from build123d import *

# Parameters (mm, degrees)
SKETCH1_W           = 13
SKETCH1_H           = 120
BOSS_EXTRUDE1_DEPTH = 9
SKETCH2_W           = 4.9
SKETCH2_H           = 6.8
BOSS_EXTRUDE2_DEPTH = 9
LPATTERN1_COUNT     = 4
LPATTERN1_PITCH     = 32
SKETCH3_W           = 4.8
SKETCH3_H           = 4.8
BOSS_EXTRUDE3_DEPTH = 9
LPATTERN2_COUNT     = 3
LPATTERN2_PITCH     = 32
SKETCH4_R           = 1.5
CUT_EXTRUDE1_DEPTH  = 9.6
CUT_EXTRUDE2_START  = -9.6
SKETCH5_R           = 1.5
CUT_EXTRUDE2_DEPTH  = 9.6
SKETCH6_W           = 13
SKETCH6_H           = 1.6
BOSS_EXTRUDE4_DEPTH = 3.7
LPATTERN3_COUNT     = 8
LPATTERN3_PITCH     = 16
SKETCH7_W           = 4.9
SKETCH7_H           = 6.8
CUT_EXTRUDE3_DEPTH  = 9
SKETCH8_W           = 4.8
SKETCH8_H           = 4.8
CUT_EXTRUDE4_DEPTH  = 9
LPATTERN4_COUNT     = 4
LPATTERN4_PITCH     = 32
LPATTERN5_COUNT     = 3
LPATTERN5_PITCH     = 32


with BuildPart() as part:
    # Sketch1 → Boss-Extrude1 (new body)
    with BuildSketch(Plane(origin=(0, 0, 0), x_dir=(1, 0, 0), z_dir=(0, 1, 0))):
        Rectangle(SKETCH1_W, SKETCH1_H)
    extrude(amount=BOSS_EXTRUDE1_DEPTH)

    # Sketch2 → Boss-Extrude2 (add)
    with BuildSketch(Plane(origin=(0, 9, 0), x_dir=(1, 0, 0), z_dir=(0, 1, 0))):
        with Locations((-8.95, 48.25183578)):
            Rectangle(SKETCH2_W, SKETCH2_H)
    boss_extrude2 = extrude(amount=-BOSS_EXTRUDE2_DEPTH)

    # LPattern1: Boss-Extrude2 ×4
    with Locations(*[(0, 0, i * LPATTERN1_PITCH) for i in range(1, LPATTERN1_COUNT)]):
        add(boss_extrude2)

    # Sketch3 → Boss-Extrude3 (add)
    with BuildSketch(Plane(origin=(0, 9, 0), x_dir=(1, 0, 0), z_dir=(0, 1, 0))):
        with Locations((-8.9, 32.256443)):
            Rectangle(SKETCH3_W, SKETCH3_H)
    boss_extrude3 = extrude(amount=-BOSS_EXTRUDE3_DEPTH)

    # LPattern2: Boss-Extrude3 ×3
    with Locations(*[(0, 0, i * LPATTERN2_PITCH) for i in range(1, LPATTERN2_COUNT)]):
        add(boss_extrude3)

    # Sketch4 → Cut-Extrude1 (cut)
    with BuildSketch(Plane.XY.offset(51.14816422)):
        with Locations((-9.5, 3)):
            Circle(SKETCH4_R)
    extrude(amount=-CUT_EXTRUDE1_DEPTH, mode=Mode.SUBTRACT)

    # Sketch5 → Cut-Extrude2 (cut)
    with BuildSketch(Plane(origin=(0, 0, -51.65183578), x_dir=(-1, 0, 0), z_dir=(0, 0, -1)).offset(CUT_EXTRUDE2_START)):
        with Locations(Location((9.5, 3, 0), (0, 0, 180))):
            Circle(SKETCH5_R)
    extrude(amount=CUT_EXTRUDE2_DEPTH, mode=Mode.SUBTRACT)

    # Sketch6 → Boss-Extrude4 (add)
    with BuildSketch(Plane(origin=(0, 9, 0), x_dir=(1, 0, 0), z_dir=(0, 1, 0))):
        with Locations((0, 57.45)):
            Rectangle(SKETCH6_W, SKETCH6_H)
        with Locations((0, 55.05)):
            Rectangle(SKETCH6_W, SKETCH6_H)
    boss_extrude4 = extrude(amount=BOSS_EXTRUDE4_DEPTH)

    # LPattern3: Boss-Extrude4 ×8
    with Locations(*[(0, 0, i * LPATTERN3_PITCH) for i in range(1, LPATTERN3_COUNT)]):
        add(boss_extrude4)

    # Sketch7 → Cut-Extrude3 (cut)
    with BuildSketch(Plane(origin=(0, 9, 0), x_dir=(1, 0, 0), z_dir=(0, 1, 0))):
        with Locations((4.05, 48.25183578)):
            Rectangle(SKETCH7_W, SKETCH7_H)
    cut_extrude3 = extrude(amount=-CUT_EXTRUDE3_DEPTH, mode=Mode.SUBTRACT)

    # Sketch8 → Cut-Extrude4 (cut)
    with BuildSketch(Plane(origin=(0, 9, 0), x_dir=(1, 0, 0), z_dir=(0, 1, 0))):
        with Locations((4.1, 32.256443)):
            Rectangle(SKETCH8_W, SKETCH8_H)
    cut_extrude4 = extrude(amount=-CUT_EXTRUDE4_DEPTH, mode=Mode.SUBTRACT)

    # LPattern4: Cut-Extrude3 ×4
    with Locations(*[(0, 0, i * LPATTERN4_PITCH) for i in range(1, LPATTERN4_COUNT)]):
        add(cut_extrude3, mode=Mode.SUBTRACT)

    # LPattern5: Cut-Extrude4 ×3
    with Locations(*[(0, 0, i * LPATTERN5_PITCH) for i in range(1, LPATTERN5_COUNT)]):
        add(cut_extrude4, mode=Mode.SUBTRACT)


solid = part.part
Input: part model. Units: mm. Frame: model coordinates. A direction names the side the tool comes from. Round coordinates to 2 decimals unless told otherwise and drop trailing zeros. Order: outer loops, then holes, each group sorted by start corner. A loop starts at its lowest first (then second) coordinate and runs counter-clockwise, first axis right, second up. Notation, with made-up numbers: (52.5, -18.75) - (100.5, -18.75) arc R21 ccw to (100.5, 13.25) - close; hole circle Ø3 at (54, -37.5). An arc over 180 degrees is marked (long way). Answer as a JSON object with one key per item and string values. Group by question number.
(1) Pin query (flat end, axial travel): P1, Ø2.5, axis at x = -9.5, y = 5, coming from the -Z side; P2, Ø4, axis at x = -9, y = 4, coming from the +Z side; P3, Ø2.5, axis at x = -9.5, y = 3, coming from the +Z side; P4, Ø3, axis at x = 2, y = 10, coming from the -Z side. Return the tip coordinate at first contact, or that it passes through.
(2) Draft query along Y for faces 5 (the face through (-10.7, 2.1, 47.8)), 6 (the face through (0, 9, 59)), 7 (the face through (4, 5, 34.144)). Return one class per face: released by +Y, released by -Y, zero draft, split by the parting line, or undercut.
(3) Cut plane B-B (x = -9.5). Count the separate pieces of the cut face and the enclosed holes in it, then the cut area to 3 significant figures.
(4) Cut plane A-A (z = -15). Return loops of the section in (x, y).
(5) Reachability of faces 1 (the face through (-6.5, 5, 7)), 2 (the face through (-11.4, 5, 48)), 3 (the face through (4, 5, 12.348)), 4 (the face through (0, 11, -42.25)) from +Z, -Z, +X, -X, +Y, -Y: full face, straight path, thin tool, end or side. Return the list, or none.
(6) Material intervals for probe 1 along Y at (x, z) = (-9.5, 49); probe 2 along X at (y, z) = (3, -48); probe 3 along X at (y, z) = (4.5, 9.5), sorted ascending. Write a range as from..to.
Here are the results:
{
 "1": {"P1": "stops at z = -51.65", "P2": "stops at z = 51.15", "P3": "stops at z = 34.14", "P4": "stops at z = -60"},
 "2": {"face 5": "undercut", "face 6": "released by +Y", "face 7": "zero draft"},
 "3": {"separate pieces": "9", "enclosed holes": "0", "area": "334 mm^2"},
 "4": {"outline": "(-11.4, 0) - (1.6, 0) - (1.6, 9) - (-11.4, 9) - close"},
 "5": {"face 1": "-X, +Y, -Y", "face 2": "+Z, -Z, -X, +Y, -Y", "face 3": "+X, +Y, -Y", "face 4": "+X, -X, +Y"},
 "6": {"probe 1": "y = 0..1.5, 4.5..9", "probe 2": "x = -11.4..-11, -8..1.6", "probe 3": "x = -6.5..6.5"}
}
